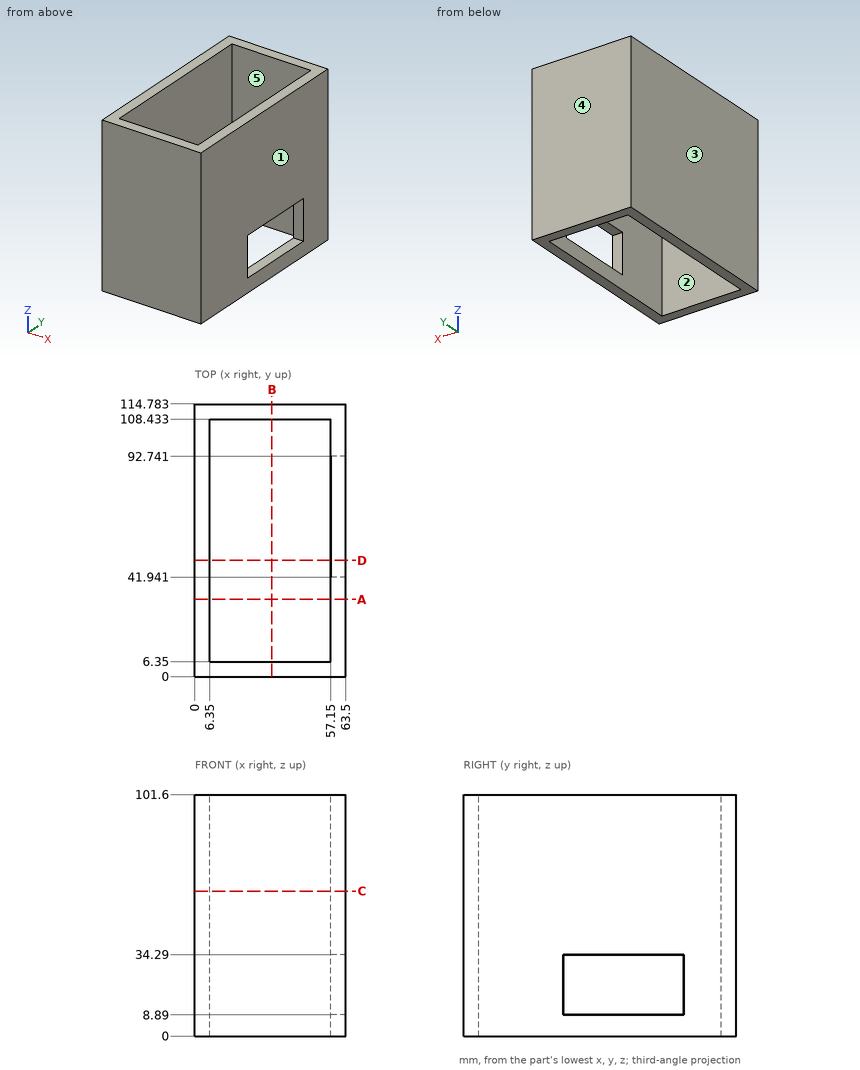
Geometry: see drawing. Coordinates: mm, zero at the bounding-box minimum. A direction names the side the tool comes from. Give positions to 0.01 mm unless a question says otherwise; leave off trailing zeros. Loops run counter-clockwise (first coordinate to the right, second up) from the corner with the lowest first, then second, coordinate; pieces in that order, holes last. Notation, with made-up numbers: M -16.75,56 L 6.25,56 A16 ccw 6.25,86 Z; hole C -35,81.25 d11. An arc over 180 degrees is marked long. Use one line per item in the form item = value.
1. First-contact query: pin 1 (5 mm diameter, centred on x = 55.5, z = 33.5, fed in from -Y). Flat tip, straight axial feed; report the tip coordinate or a pass-through.
Numbers:
pin_1 = 0
2. Section query C-C, the plane z = 61. Return the cut outline in (x, y).
Numbers:
outline = M 0,0 L 63.5,0 L 63.5,114.78 L 0,114.78 Z; hole M 6.35,6.35 L 57.15,6.35 L 57.15,108.43 L 6.35,108.43 Z
3. Section query B-B, the plane x = 32.5. Return the cut outline in (y, z), and give its area (3 significant figures).
Numbers:
outline = M 0,0 L 6.35,0 L 6.35,101.6 L 0,101.6 Z; M 108.43,0 L 114.78,0 L 114.78,101.6 L 108.43,101.6 Z
area = 1,290 mm²
4. Section query D-D, the plane y = 49. Return the cut outline in (x, z).
Numbers:
outline = M 0,0 L 6.35,0 L 6.35,101.6 L 0,101.6 Z; M 57.15,0 L 63.5,0 L 63.5,8.89 L 57.15,8.89 Z; M 57.15,34.29 L 63.5,34.29 L 63.5,101.6 L 57.15,101.6 Z
5. Line query: L1, parallel to Y at x = 10, z = 21; L2, parallel to X at y = 98, z = 14; L3, parallel to X at y = 65, z = 25. Output: solid intervals per line, ascending.
Numbers:
L1 = 0 to 6.35, 108.43 to 114.78
L2 = 0 to 6.35, 57.15 to 63.5
L3 = 0 to 6.35
6. Section query A-A, the plane y = 32.5. Return the cut outline in (x, z).
Numbers:
outline = M 0,0 L 6.35,0 L 6.35,101.6 L 0,101.6 Z; M 57.15,0 L 63.5,0 L 63.5,101.6 L 57.15,101.6 Z
7. Reachability of the marked faces 1 and 2 from +Z, -Z, +X, -X, +Y, -Y: full face, straight path, thin tool, end or side. Return the list, or none.
Numbers:
face_1 = +Z, -Z, +X, +Y, -Y
face_2 = +Z, -Z
8. Pull-direction query (X, two-part tool) for the marked faces 3, 4 and 5; classes: released by +X, released by -X, zero draft, split by the parting line, or undercut.
Numbers:
face_3 = released by -X
face_4 = zero draft
face_5 = undercut
